The listing builds one solid part. Answer for the finished solid, in the listing's coordinates (mm). Round coordinates to 2 decimals unless told otherwise and drop trailing zeros. Order: outer loops, then holes, each group sorted by start corner. A loop starts at its lowest first (then second) coordinate and runs counter-clockwise, first axis right, second up. Notation, with made-up numbers: (2.25, 1.5) - (52.25, 1.5) arc R20 ccw to (52.25, 28.5) - close; hole circle Ø3 at (74, -4). An arc over 180 degrees is marked (long way). Write item = value, one per line.
from build123d import *

# Parameters (mm, degrees)
EXTRUDE1_DEPTH = 4.5
FILLET1_R      = 0.5


with BuildPart() as part:
    # Sketch1 → Extrude1 (new body)
    with BuildSketch(Plane.XY):
        with BuildLine():
            ThreePointArc((-0.746559936, 18.690444938), (1.504276061, -0.190220828), (7.658793849, -18.180988273))
            ThreePointArc((7.658793849, -18.180988273), (7.66003149, -20.530722722), (5.866174119, -22.048395034))
            ThreePointArc((5.866174119, -22.048395034), (2.294255729, -21.716159254), (-0.170136467, -19.109292801))
            ThreePointArc((-0.170136467, -19.109292801), (-5.883088092, -0.625489951), (-7.918665293, 18.613668282))
            ThreePointArc((-7.918665293, 18.613668282), (-4.370906261, 22.229264553), (-0.746559936, 18.690444938))
        make_face()
    extrude(amount=EXTRUDE1_DEPTH)

    # Fillet1
    fillet1_edges = [part.edges().sort_by_distance(p)[0] for p in [
        (2.294255729, -21.716159254, 4.5),
        (7.66003149, -20.530722722, 4.5),
        (1.504276061, -0.190220828, 4.5),
        (-4.370906261, 22.229264553, 4.5),
        (-5.883088092, -0.625489951, 4.5),
    ]]
    fillet(fillet1_edges, radius=FILLET1_R)


solid = part.part
Q1. Find the intervals of material crossed by line 1 (X direction, y = 2.5, z = 3.3); line 2 (X direction, y = -19, z = 2.45); line 3 (Y direction, x = 6.5, z = 1.7), in increasing order. Write a range as from..to.
Model answer:
line_1 = -6.47..0.93
line_2 = -0.22..7.9
line_3 = -21.79..-15.58
Q2. A flat-ended cylindrical pin translates along its axis: P1, Ø2, axis at y = -10.5, z = 1.5, coming from the +X side. Find the tip coordinate at first contact, or state that the pin passes through.
Model answer:
P1 = 4.87
Q3. Section A-A on z = 1.45 is taken. Determine the outline of the cut face in (x, y).
Model answer:
outline = (-7.92, 18.61) arc R99.7 ccw to (-0.17, -19.11) arc R5.09 ccw to (5.87, -22.05) arc R2.79 ccw to (7.66, -18.18) arc R90.3 cw to (-0.75, 18.69) arc R3.59 ccw to start
